Geometry: final body of the model. Coordinates: model frame, mm. Face numbers are marked on the shaded views. A direction names the side the tool comes from. Round coordinates to 2 decimals unless told otherwise and drop trailing zeros. Order: outer loops, then holes, each group sorted by start corner. A loop starts at its lowest first (then second) coordinate and runs counter-clockwise, first axis right, second up. Notation, with made-up numbers: M 84.5,78.25 L 122.5,78.25 A26 ccw 122.5,93.25 Z; hole C 64,9.5 d3. An arc over 180 degrees is marked long. Put each result on its own line as item: value. Start each with the question number.
1) Section A-A, the plane z = -12.7. Return loops of the section in (x, y).
2) Draft query along X for the marked faces 4, 5 and 6. Return one class per face: pulls with the +X half, pulls with the -X half, needs draft (parallel to the pull), parting line crosses it, or undercut.
3) Access query for the marked faces 1, 2 and 3. Directions: +Z, -Z, +X, -X, +Y, -Y. A direction counts if a zero-diameter tool reaches every point of the face in a straight line with its end or side. Return the directions, or none.
4) Material intervals for probe 1 along X at (y, z) = (2.15, 0); probe 2 along X at (y, z) = (3.75, -12.7); probe 3 along Z at (x, y) = (8, 2.7), sorted ascending. Write a range as [from, to].
5) Section C-C, the plane y = 1.3. Count the separate pieces of the cut face and the enclosed holes in it, then the cut area to 3 significant figures.
6) Section D-D, the plane x = -11.5. Return loops of the section in (y, z), then the cut area to 3 significant figures.
7) First-contact query: P1, Ø3, axis at x = -10.5, y = 4.5, coming from the +Z side; P2, Ø1.8, axis at x = -10.5, y = 3.5, coming from the -Z side. Flat tips, straight axial feed; report the tip coordinate or a pass-through.
8) Section B-B, the plane x = -19.05. Return loops of the section in (y, z).
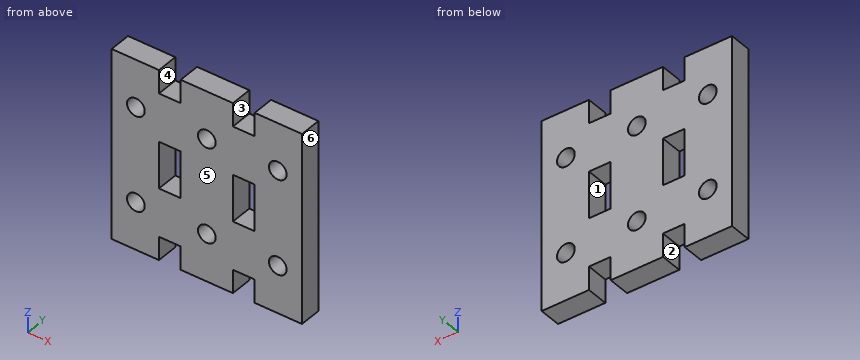
from build123d import *

# Parameters (mm, degrees)
SKETCH1_W           = 5.842
SKETCH1_H           = 12.5
BOSS_EXTRUDE1_DEPTH = 5.842
SKETCH2_R           = 2.38125
CUT_EXTRUDE1_DEPTH  = 37.500628488


with BuildPart() as part:
    # Sketch1 → Boss-Extrude1 (new body)
    with BuildSketch(Plane(origin=(0, 0, 0), x_dir=(1, 0, 0), z_dir=(0, 1, 0))):
        Polygon((7.012, -25.4), (-7.012, -25.4), (-7.012, -19.15), (-12.854, -19.15), (-12.854, -25.4), (-25.554, -25.4), (-25.554, 25.4), (-12.854, 25.4), (-12.854, 19.15), (-7.012, 19.15), (-7.012, 25.4), (7.012, 25.4), (7.012, 19.15), (12.854, 19.15), (12.854, 25.4), (25.554, 25.4), (25.554, -25.4), (12.854, -25.4), (12.854, -19.15), (7.012, -19.15), align=None)
        with Locations((-9.933, 0)):
            Rectangle(SKETCH1_W, SKETCH1_H, mode=Mode.SUBTRACT)
        with Locations((9.933, 0)):
            Rectangle(SKETCH1_W, SKETCH1_H, mode=Mode.SUBTRACT)
    extrude(amount=BOSS_EXTRUDE1_DEPTH)

    # Sketch2 → Cut-Extrude1 (cut, through all)
    with BuildSketch(Plane(origin=(0, 5.842, 0), x_dir=(1, 0, 0), z_dir=(0, 1, 0))):
        with Locations(Location((0, -12.7, 0), (0, 0, 270))):
            Circle(SKETCH2_R)
        with Locations(Location((0, 12.7, 0), (0, 0, 90))):
            Circle(SKETCH2_R)
        with Locations(Location((19.05, 12.7, 0), (0, 0, 270))):
            Circle(SKETCH2_R)
        with Locations(Location((19.05, -12.7, 0), (0, 0, 90))):
            Circle(SKETCH2_R)
        with Locations(Location((-19.05, 12.7, 0), (0, 0, 90))):
            Circle(SKETCH2_R)
        with Locations(Location((-19.05, -12.7, 0), (0, 0, 270))):
            Circle(SKETCH2_R)
    extrude(amount=-CUT_EXTRUDE1_DEPTH, mode=Mode.SUBTRACT)


solid = part.part
Result sheet:
1. outline: M -25.55,0 L -21.43,0 L -21.43,5.84 L -25.55,5.84 Z; M -16.67,0 L -2.38,0 L -2.38,5.84 L -16.67,5.84 Z; M 2.38,0 L 16.67,0 L 16.67,5.84 L 2.38,5.84 Z; M 21.43,0 L 25.55,0 L 25.55,5.84 L 21.43,5.84 Z
2. face 4: undercut
2. face 5: needs draft
2. face 6: pulls with the +X half
3. face 1: +Y, -Y
3. face 2: -Z, +Y, -Y
3. face 3: +Z, +Y, -Y
4. probe 1: x = [-25.55, -12.85], [-7.01, 7.01], [12.85, 25.55]
4. probe 2: x = [-25.55, -21.43], [-16.67, -2.38], [2.38, 16.67], [21.43, 25.55]
4. probe 3: z = [-19.15, -6.25], [6.25, 19.15]
5. separate pieces: 1
5. enclosed holes: 8
5. area: 2,200 mm2
6. outline: M 0,-19.15 L 5.84,-19.15 L 5.84,-6.25 L 0,-6.25 Z; M 0,6.25 L 5.84,6.25 L 5.84,19.15 L 0,19.15 Z
6. area: 151 mm2
7. P1: stops at z = 19.15
7. P2: stops at z = -19.15
8. outline: M 0,-25.4 L 5.84,-25.4 L 5.84,-15.08 L 0,-15.08 Z; M 0,-10.32 L 5.84,-10.32 L 5.84,10.32 L 0,10.32 Z; M 0,15.08 L 5.84,15.08 L 5.84,25.4 L 0,25.4 Z
